Could you check a few things on this model? Use its own coordinates, in mm. A direction names the side the tool comes from. Round coordinates to 2 decimals unless told otherwise and drop trailing zeros. Order: outer loops, then holes, each group sorted by start corner. A loop starts at its lowest first (then second) coordinate and runs counter-clockwise, first axis right, second up. Notation, with made-up numbers: M 67.5,67 L 81.5,67 A35 ccw 81.5,104 Z; hole C 30.5,22 d3. An arc over 180 degrees is marked long. Write each question's results on one line, items separated by ' | '. Start each with the question number.
1. Suppose I cut it at A-A on z = -27. Write out the boundary of the cut face in (x, y).
2. I'm going to push flat-ended pins straight in: pin 1 (2.5 mm diameter, centred on x = -25, z = 13, fed in from +Y); pin 2 (1.5 mm diameter, centred on x = 19.05, z = -36.7, fed in from -Y); pin 3 (2.5 mm diameter, centred on x = 9, y = 4.5, fed in from +Z); pin 4 (16 mm diameter, centred on x = 8, z = -7.5, fed in from +Y). Where does each tip first touch, or does it pass through?
3. We'd pull the mould along Z, two halves only. Please class faces 1 (the flat face through (25, 5, -36.9)), 2 (the flat face through (5, 4, -41.7)), 3 (the flat face through (25, 4, 17.63)), 4 (the flat face through (28, 7.32, -3)): released by +Z, released by -Z, zero draft, split by the parting line, or undercut.
4. Suppose I cut it at C-C on x = 6.5. Write out the boundary of the cut face in (y, z), and give its area (3 significant figures).
5. Please list where these lines run through material, in increasing order: L1, parallel to X at y = 1, z = 34.8; L2, parallel to X at y = 1.95, z = -36.7; L3, parallel to Z at x = 19.05, y = 1.35.
6. Suppose I cut it at D-D on z = -17. Write out the boundary of the cut face in (x, y).
7. For faces 5 (the flat face through (27, 4, -39.1)), 6 (the cylindrical face through (22.55, 2.64, 15.18)), 7 (the flat face through (-25, 4, 11.69)), which set-ups out of +Z, -Z, +X, -X, +Y, -Y let a thin tool reach every point of the face, with its end or its side?
8. Suppose I cut it at B-B on y = 1. Give the number of separate pieces and of enclosed holes in the cut face, and give its area (3 significant figures).
from build123d import *

# Parameters (mm, degrees)
BOSS_EXTRUDE1_DEPTH = 2.2
EXTRUDE_THIN1_DEPTH = 5.12
BOSS_EXTRUDE2_DEPTH = 3
SKETCH6_R           = 1.25
SKETCH6_R_2         = 1.5
CUT_EXTRUDE1_DEPTH  = 8.32


with BuildPart() as part:
    # Sketch1 → Boss-Extrude1 (new body)
    with BuildSketch(Plane(origin=(0, 0, 0), x_dir=(1, 0, 0), z_dir=(0, 1, 0))):
        Polygon((-15.25, 39.1), (-12.65, 41.7), (22.15, 41.7), (24.75, 39.1), (28.75, 39.1), (28.75, -39.1), (-28.75, -39.1), (-28.75, 39.1), align=None)
    extrude(amount=BOSS_EXTRUDE1_DEPTH)

    # Sketch3 → Extrude-Thin1 (add)
    with BuildSketch(Plane(origin=(0, 2.2, 0), x_dir=(1, 0, 0), z_dir=(0, 1, 0))):
        Polygon((-28.75, 39.1), (-15.25, 39.1), (-12.65, 41.7), (22.15, 41.7), (24.75, 39.1), (28.75, 39.1), (28.75, -31.1), (-28.75, -31.1), align=None)
        Polygon((-26.55, 36.9), (-14.338730163, 36.9), (-11.738730163, 39.5), (21.238730163, 39.5), (23.838730163, 36.9), (26.55, 36.9), (26.55, -28.9), (-26.55, -28.9), align=None, mode=Mode.SUBTRACT)
    extrude(amount=EXTRUDE_THIN1_DEPTH)

    # Sketch4 → Boss-Extrude2 (add)
    with BuildSketch(Plane(origin=(0, 2.2, 0), x_dir=(1, 0, 0), z_dir=(0, 1, 0))):
        with BuildLine():
            Line((-11.08, 39.5), (-6.68, 39.5))
            Line((-6.68, 39.5), (-6.68, 36.7))
            ThreePointArc((-6.68, 36.7), (-8.88, 34.5), (-11.08, 36.7))
            Line((-11.08, 36.7), (-11.08, 39.5))
        make_face()
        with BuildLine():
            Line((16.85, 39.5), (21.25, 39.5))
            Line((21.25, 39.5), (21.25, 36.7))
            ThreePointArc((21.25, 36.7), (19.05, 34.5), (16.85, 36.7))
            Line((16.85, 36.7), (16.85, 39.5))
        make_face()
        with BuildLine():
            Line((26.55, -12.83), (23.8, -12.83))
            ThreePointArc((23.8, -12.83), (21.4, -15.23), (23.8, -17.63))
            Line((23.8, -17.63), (26.55, -17.63))
            Line((26.55, -17.63), (26.55, -12.83))
        make_face()
        with BuildLine():
            Line((-26.55, -11.69), (-24.086432316, -11.69))
            ThreePointArc((-24.086432316, -11.69), (-21.686432316, -14.09), (-24.086432316, -16.49))
            Line((-24.086432316, -16.49), (-26.55, -16.49))
            Line((-26.55, -16.49), (-26.55, -11.69))
        make_face()
    extrude(amount=BOSS_EXTRUDE2_DEPTH)

    # Sketch6 → Cut-Extrude1 (cut, through all)
    with BuildSketch(Plane(origin=(0, 7.32, 0), x_dir=(1, 0, 0), z_dir=(0, 1, 0))):
        with Locations((-8.88, 36.7)):
            Circle(SKETCH6_R)
        with Locations((19.05, 36.7)):
            Circle(SKETCH6_R)
        with Locations((23.8, -15.23)):
            Circle(SKETCH6_R)
        with Locations((-24.086432316, -14.09)):
            Circle(SKETCH6_R)
        with Locations((-19.15, 27)):
            Circle(SKETCH6_R_2)
        with Locations((19.25, 27)):
            Circle(SKETCH6_R_2)
        with Locations((-24.45, -34.8)):
            Circle(SKETCH6_R_2)
        with Locations((24.55, -34.8)):
            Circle(SKETCH6_R_2)
    extrude(amount=-CUT_EXTRUDE1_DEPTH, mode=Mode.SUBTRACT)


solid = part.part
Filled sheet:
1) outline: M -28.75,0 L -20.65,0 L -20.65,2.2 L -26.55,2.2 L -26.55,7.32 L -28.75,7.32 Z; M -17.65,0 L 17.75,0 L 17.75,2.2 L -17.65,2.2 Z; M 20.75,0 L 28.75,0 L 28.75,7.32 L 26.55,7.32 L 26.55,2.2 L 20.75,2.2 Z
2) pin 1: stops at y = 5.2 | pin 2: passes through | pin 3: stops at z = 31.1 | pin 4: stops at y = 2.2
3) face 1: undercut | face 2: released by -Z | face 3: undercut | face 4: zero draft
4) outline: M 0,-41.7 L 7.32,-41.7 L 7.32,-39.5 L 2.2,-39.5 L 2.2,28.9 L 7.32,28.9 L 7.32,31.1 L 2.2,31.1 L 2.2,39.1 L 0,39.1 Z | area: 200 mm^2
5) L1: x = -28.75 to -25.95, -22.95 to 23.05, 26.05 to 28.75 | L2: x = -28.75 to -10.13, -7.63 to 17.8, 20.3 to 28.75 | L3: z = -41.7 to -37.95, -35.45 to -28.49, -25.51 to 39.1
6) outline: M -28.75,0 L 28.75,0 L 28.75,7.32 L 26.55,7.32 L 26.55,2.2 L -26.55,2.2 L -26.55,7.32 L -28.75,7.32 Z
7) face 5: -Z, +X, +Y, -Y | face 6: +Y, -Y | face 7: +Y
8) separate pieces: 1 | enclosed holes: 8 | area: 4,550 mm^2
